Autodesk Inventor part; units mm, degrees
ref_plane "YZ Plane" through (0, 0, 0) normal (1, 0, 0) x (0, 1, 0)
ref_plane "XZ Plane" through (0, 0, 0) normal (0, 1, 0) x (-1, 0, 0)
ref_plane "XY Plane" through (0, 0, 0) normal (0, 0, 1) x (1, 0, 0)
sketch "Sketch1" plane through (0, 0, 0) normal (0, 1, 0) x (-1, 0, 0)
  line L0 (-10, 85) -> (10, 85)
  line L1 (10, 85) -> (10, -85)
  line L2 (10, -85) -> (-10, -85)
  line L3 (-10, -85) -> (-10, 85)
  line L4 (-10, 85) -> (10, -85) construction
  line L5 (10, 85) -> (-10, -85) construction
  point P0 (0, 0)
  dimension "d0" = 170
  dimension "d1" = 20
extrude "Extrusion1" add sketch "Sketch1" along normal blind 5
sketch "Sketch2" plane through (0, 5, 0) normal (0, 1, 0) x (1, 0, 0)
  line L0 (0, 0) -> (10.5, 0)
  line L1 (6, -37.5) -> (15, -37.5)
  line L2 (15, -37.5) -> (15, 37.5)
  line L3 (15, 37.5) -> (6, 37.5)
  line L4 (6, 37.5) -> (6, -37.5)
  line L5 (6, -37.5) -> (15, 37.5) construction
  line L6 (15, -37.5) -> (6, 37.5) construction
  line L7 (10, -85) -> (10, 85)
  point P0 (10, 37.5)
  point P1 (10, -37.5)
  dimension "d4" = 5
  dimension "d5" = 75
extrude "Extrusion2" add sketch "Sketch2" against normal blind 5 contours L7 L3 L2 L1
mirror "Mirror1" about plane through (0, 0, 0) normal (1, 0, 0) of "Extrusion2"
properties part number "Gel wall"
The model under review builds one solid part; all positions refer to its coordinate system, in mm. A direction names the side the tool comes from. Round coordinates to 2 decimals unless told otherwise and drop trailing zeros. Order: outer loops, then holes, each group sorted by start corner. A loop starts at its lowest first (then second) coordinate and runs counter-clockwise, first axis right, second up. Notation, with made-up numbers: (50, 85.5) -> (93, 85.5) arc R22 cw to (93, 91.5) -> close; hole circle Ø9 at (-38, 28). An arc over 180 degrees is marked (long way). Write item = value, one per line. Start each with the question number.
Item 1: Consider section A-A on y = 2.3. Write out the cut boundary in (x, z).
Item 2: Consider section B-B on z = 70. Write out the cut boundary in (x, y), plus the area to 3 significant figures.
Item 3: For faces 1 (the face through (10, 2, 61)), 2 (the face through (13, 3, -37.5)), 3 (the face through (0, 5, 1)), 4 (the face through (-10, 2, 62)), 5 (the face through (0, 0, 1)), list the 3-axis set-ups (+Z, -Z, +X, -X, +Y, -Y) from which the entire face can be reached by the end or side of a thin tool; tool diameter is ignored.
Item 4: Consider section C-C on x = 11.75. Write out the cut boundary in (y, z), plus the area to 3 significant figures.
Item 5: For line 1 along Z through (x, y) = (-11, 1.2); line 2 along X through (y, z) = (1.05, 38.5), list the stretches that pass through material, from the lowest coordinate up.
Item 6: Clearance check with a flat-ended pin moving along its axis: pin 1 Ø2.5 at (x, y) = (-13.5, 1.5) entering from -Z. State where the tip first meets the part, or that it passes through.
Item 7: Mouldability with a two-part tool opening along Z and no side actions: class faces 6 (the face through (-10, 2, -61)), 7 (the face through (-12, 3, -37.5)), 8 (the face through (-13, 3, 37.5)) as released by +Z, released by -Z, zero draft, split by the parting line, or undercut.
Conclusion:
q1.outline = (-15, -37.5) -> (-10, -37.5) -> (-10, -85) -> (10, -85) -> (10, -37.5) -> (15, -37.5) -> (15, 37.5) -> (10, 37.5) -> (10, 85) -> (-10, 85) -> (-10, 37.5) -> (-15, 37.5) -> close
q2.outline = (-10, 0) -> (10, 0) -> (10, 5) -> (-10, 5) -> close
q2.area = 100 mm2
q3.face_1 = +Z, +X, +Y, -Y
q3.face_2 = -Z, +X, +Y, -Y
q3.face_3 = +Z, -Z, +X, -X, +Y
q3.face_4 = +Z, -X, +Y, -Y
q3.face_5 = +Z, -Z, +X, -X, -Y
q4.outline = (0, -37.5) -> (5, -37.5) -> (5, 37.5) -> (0, 37.5) -> close
q4.area = 375 mm2
q5.line_1 = -37.5 to 37.5
q5.line_2 = -10 to 10
q6.pin_1 = -37.5
q7.face_6 = zero draft
q7.face_7 = released by -Z
q7.face_8 = released by +Z
